```python
from build123d import *

# Parameters (mm, degrees)
BOSS_EXTRUDE1_DEPTH  = 2.5
FILLET1_R            = 5
BOSS_EXTRUDE2_DEPTH  = 9.8
CUT_EXTRUDE1_DEPTH   = 9.8
CUT_EXTRUDE2_DEPTH   = 89.657557489
BOSS_EXTRUDE3_DEPTH  = 11.7
MIRROR4_COPY_1_DEPTH = 11.7
SKETCH8_W            = 22.2
SKETCH8_H            = 28.2
CUT_EXTRUDE3_DEPTH   = 10


with BuildPart() as part:
    # Sketch1 → Boss-Extrude1 (new body)
    with BuildSketch(Plane(origin=(0, 0, 0), x_dir=(1, 0, 0), z_dir=(0, 1, 0))):
        with BuildLine():
            Line((-46.5, 30), (46.5, 30))
            ThreePointArc((46.5, 30), (50.035533906, 28.535533906), (51.5, 25))
            Line((51.5, 25), (51.5, -25))
            ThreePointArc((51.5, -25), (50.035533906, -28.535533906), (46.5, -30))
            Line((46.5, -30), (-46.5, -30))
            ThreePointArc((-46.5, -30), (-50.035533906, -28.535533906), (-51.5, -25))
            Line((-51.5, -25), (-51.5, 25))
            ThreePointArc((-51.5, 25), (-50.035533906, 28.535533906), (-46.5, 30))
        make_face()
    extrude(amount=BOSS_EXTRUDE1_DEPTH)

    # Fillet1
    # the kernel refuses this fillet: 5 mm, written as the material it takes off along each edge
    with BuildSketch(Plane(origin=(-46.5, 2.5, -25), x_dir=(-1, 0, 0), z_dir=(0, 0, 1))) as fillet1_piece_1:
        with BuildLine():
            CenterArc((0.669872981, 5), FILLET1_R, 270, 60)
            Line((0.669872981, 0), (0.669872981, -0.1))
            Line((0.669872981, -0.1), (5, -0.1))
            Line((5, -0.1), (5.1, 0))
            ThreePointArc((5.1, 0), (5.1, 1.25), (5.08660254, 2.45))
            Line((5.08660254, 2.45), (5, 2.5))
        make_face()
    revolve(axis=Axis((-46.5, 2.5, -25), (0, -1, 0)), revolution_arc=90, mode=Mode.SUBTRACT)
    with BuildSketch(Plane(origin=(-46.5, 2.5, -30), x_dir=(0, -1, 0), z_dir=(1, 0, 0)), Plane(origin=(46.5, 2.5, 30), x_dir=(0, -1, 0), z_dir=(-1, 0, 0))) as fillet1_piece_2:
        with BuildLine():
            CenterArc((5, -4.330127019), FILLET1_R, 120, 60)
            Line((0, -4.330127019), (-0.1, -4.330127019))
            Line((-0.1, -4.330127019), (-0.1, 0))
            Line((-0.1, 0), (0, 0.1))
            ThreePointArc((0, 0.1), (1.25, 0.1), (2.45, 0.08660254))
            Line((2.45, 0.08660254), (2.5, 0))
        make_face()
    extrude(amount=93, mode=Mode.SUBTRACT)
    with BuildSketch(Plane(origin=(46.5, 2.5, -25), x_dir=(0, 0, -1), z_dir=(-1, 0, 0))) as fillet1_piece_3:
        with BuildLine():
            CenterArc((0.669872981, 5), FILLET1_R, 270, 60)
            Line((0.669872981, 0), (0.669872981, -0.1))
            Line((0.669872981, -0.1), (5, -0.1))
            Line((5, -0.1), (5.1, 0))
            ThreePointArc((5.1, 0), (5.1, 1.25), (5.08660254, 2.45))
            Line((5.08660254, 2.45), (5, 2.5))
        make_face()
    revolve(axis=Axis((46.5, 2.5, -25), (0, -1, 0)), revolution_arc=90, mode=Mode.SUBTRACT)
    with BuildSketch(Plane(origin=(51.5, 2.5, -25), x_dir=(0, -1, 0), z_dir=(0, 0, 1)), Plane(origin=(-51.5, 2.5, 25), x_dir=(0, -1, 0), z_dir=(0, 0, -1))) as fillet1_piece_4:
        with BuildLine():
            CenterArc((5, -4.330127019), FILLET1_R, 120, 60)
            Line((0, -4.330127019), (-0.1, -4.330127019))
            Line((-0.1, -4.330127019), (-0.1, 0))
            Line((-0.1, 0), (0, 0.1))
            ThreePointArc((0, 0.1), (1.25, 0.1), (2.45, 0.08660254))
            Line((2.45, 0.08660254), (2.5, 0))
        make_face()
    extrude(amount=50, mode=Mode.SUBTRACT)
    with BuildSketch(Plane(origin=(46.5, 2.5, 25), x_dir=(1, 0, 0), z_dir=(0, 0, -1))) as fillet1_piece_5:
        with BuildLine():
            CenterArc((0.669872981, 5), FILLET1_R, 270, 60)
            Line((0.669872981, 0), (0.669872981, -0.1))
            Line((0.669872981, -0.1), (5, -0.1))
            Line((5, -0.1), (5.1, 0))
            ThreePointArc((5.1, 0), (5.1, 1.25), (5.08660254, 2.45))
            Line((5.08660254, 2.45), (5, 2.5))
        make_face()
    revolve(axis=Axis((46.5, 2.5, 25), (0, -1, 0)), revolution_arc=90, mode=Mode.SUBTRACT)
    with BuildSketch(Plane(origin=(-46.5, 2.5, 25), x_dir=(0, 0, 1), z_dir=(1, 0, 0))) as fillet1_piece_6:
        with BuildLine():
            CenterArc((0.669872981, 5), FILLET1_R, 270, 60)
            Line((0.669872981, 0), (0.669872981, -0.1))
            Line((0.669872981, -0.1), (5, -0.1))
            Line((5, -0.1), (5.1, 0))
            ThreePointArc((5.1, 0), (5.1, 1.25), (5.08660254, 2.45))
            Line((5.08660254, 2.45), (5, 2.5))
        make_face()
    revolve(axis=Axis((-46.5, 2.5, 25), (0, -1, 0)), revolution_arc=90, mode=Mode.SUBTRACT)

    # Sketch2 → Boss-Extrude2 (add)
    with BuildSketch(Plane.XZ):
        Polygon((-36.2, 28.5), (-24.5, 28.5), (-24.5, 26.5), (-29.35, 26.5), (-29.35, 20.5), (-31.35, 20.5), (-31.35, 26.5), (-36.2, 26.5), align=None)
        Polygon((48.225, -3.282847821), (46.225, -3.282847821), (46.225, -0.999790058), (40.225, -0.999790058), (40.225, 1), (46.225, 1), (46.225, 3.417152179), (48.225, 3.417152179), align=None)
        Polygon((24.5, 28.5), (36.2, 28.5), (36.2, 26.5), (31.35, 26.5), (31.35, 20.5), (29.35, 20.5), (29.35, 26.5), (24.5, 26.5), align=None)
        Polygon((24.5, -26.5), (29.35, -26.5), (29.35, -20.5), (31.35, -20.5), (31.35, -26.5), (36.2, -26.5), (36.2, -28.5), (24.5, -28.5), align=None)
        Polygon((-36.2, -28.5), (-24.5, -28.5), (-24.5, -26.5), (-29.35, -26.5), (-29.35, -20.5), (-31.35, -20.5), (-31.35, -26.5), (-36.2, -26.5), align=None)
        Polygon((-48.225, 3.417152179), (-46.225, 3.417152179), (-46.225, 1), (-40.225, 1), (-40.225, -0.999790058), (-46.225, -0.999790058), (-46.225, -3.282847821), (-48.225, -3.282847821), align=None)
    extrude(amount=BOSS_EXTRUDE2_DEPTH)

    # Sketch4 → Cut-Extrude1 (cut)
    with BuildSketch(Plane(origin=(0, 0, -0.999790058), x_dir=(-1, 0, 0), z_dir=(0, 0, -1))):
        Polygon((40.225, 0), (46.225, -9.8), (40.225, -9.8), align=None)
    cut_extrude1 = extrude(amount=-CUT_EXTRUDE1_DEPTH, mode=Mode.SUBTRACT)

    # Mirror1: Cut-Extrude1 across plane
    add(cut_extrude1.mirror(Plane(origin=(0, 0, 0), x_dir=(0, 0, 1), z_dir=(1, 0, 0))), mode=Mode.SUBTRACT)

    # Sketch5 → Cut-Extrude2 (cut, through all)
    with BuildSketch(Plane.ZY.offset(31.35)):
        Polygon((-26.5, -9.8), (-20.5, 0), (-20.5, -9.8), align=None)
    cut_extrude2 = extrude(amount=-CUT_EXTRUDE2_DEPTH, mode=Mode.SUBTRACT)

    # Mirror2: Cut-Extrude2 across plane
    add(cut_extrude2.mirror(Plane.XY), mode=Mode.SUBTRACT)

    # Sketch6 → Boss-Extrude3 (add)
    with BuildSketch(Plane(origin=(36.2, 0, 0), x_dir=(0, 0, -1), z_dir=(1, 0, 0))):
        Polygon((-28.5, -3), (-28.5, -7.5), (-30, -3.726144837), align=None)
    boss_extrude3 = extrude(amount=-BOSS_EXTRUDE3_DEPTH)

    # Mirror3: Boss-Extrude3 across plane
    add(boss_extrude3.mirror(Plane(origin=(0, 0, 0), x_dir=(0, 0, 1), z_dir=(1, 0, 0))))

    # Mirror4: Boss-Extrude3 across plane
    add(boss_extrude3.mirror(Plane.XY))

    # Mirror4 copy 1 sketch → Mirror4 copy 1 (add)
    with BuildSketch(Plane.ZY.offset(36.2)):
        Polygon((-28.5, -3), (-28.5, -7.5), (-30, -3.726144837), align=None)
    extrude(amount=-MIRROR4_COPY_1_DEPTH)

    # Sketch8 → Cut-Extrude3 (cut)
    with BuildSketch(Plane.XZ):
        with Locations((-21.1, 0)):
            Rectangle(SKETCH8_W, SKETCH8_H)
        with Locations((21.1, 0)):
            Rectangle(SKETCH8_W, SKETCH8_H)
    extrude(amount=-CUT_EXTRUDE3_DEPTH, mode=Mode.SUBTRACT)


solid = part.part
```
Check sheet for the modelled part. Datum: model origin and axes. Units: mm. A direction names the side the tool comes from. Round coordinates to 2 decimals unless told otherwise and drop trailing zeros. Order: outer loops, then holes, each group sorted by start corner. A loop starts at its lowest first (then second) coordinate and runs counter-clockwise, first axis right, second up. Notation, with made-up numbers: M -22.5,89 L 5.5,89 A18 ccw 5.5,99 Z; hole C -23,29 d8. An arc over 180 degrees is marked long. Answer in a Markdown table with one row per item.
(1) Set-up check for faces 4 (the flat face through (31.35, -3, -25)), 5 (the flat face through (-44, -4, 1)), 6 (the flat face through (30, -1, -28.5)), 7 (the flat face through (24.5, -5, 28)): record each of +Z, -Z, +X, -X, +Y, -Y from which the full face is reachable in a straight line by a thin tool's end or side.
Findings:
| item | result |
|---|---|
| face 4 | +X, -Y |
| face 5 | +Z, -Y |
| face 6 | -Z, +X, -X |
| face 7 | +Z, -Z, -Y |
(2) Section check D-D on y = -5.5. Give the number of separate pieces and of enclosed holes in the cut face, plus the area to 3 significant figures.
Findings:
| item | result |
|---|---|
| separate pieces | 6 |
| enclosed holes | 0 |
| area | 189 mm^2 |
(3) Section check C-C on x = 35. Record the boundary of the cut face in (y, z).
Findings:
| item | result |
|---|---|
| outline | M -9.8,-28.5 L -7.5,-28.5 L -3.73,-30 L -3,-28.5 L 0,-28.5 L 0,-30 A5 ccw 2.5,-25.67 L 2.5,25.67 A5 ccw 0,30 L 0,28.5 L -3,28.5 L -3.73,30 L -7.5,28.5 L -9.8,28.5 L -9.8,26.5 L 0,26.5 L 0,-26.5 L -9.8,-26.5 Z |
(4) Section check B-B on x = -17. Record the boundary of the cut face in (y, z).
Findings:
| item | result |
|---|---|
| outline | M 0,-30 A5 ccw 2.5,-25.67 L 2.5,-14.1 L 0,-14.1 Z; M 0,14.1 L 2.5,14.1 L 2.5,25.67 A5 ccw 0,30 Z |
(5) Gauge pin test, flat ends, axial feed: pin 1 (0.8 mm diameter, centred on y = 1, z = -7, fed in from +X); pin 2 (5.5 mm diameter, centred on x = -26, y = -6.5, fed in from -Z); pin 3 (5 mm diameter, centred on y = 0.5, z = 3.5, fed in from -X). Record the tip position at first contact, or that the pin passes through.
Findings:
| item | result |
|---|---|
| pin 1 | stops at x = 51.09 |
| pin 2 | stops at z = -29.99 |
| pin 3 | stops at x = -51.5 |
(6) Section check A-A on z = 7. Record the boundary of the cut face in (x, y).
Findings:
| item | result |
|---|---|
| outline | M -51.5,0 L -32.2,0 L -32.2,2.5 L -47.17,2.5 A5 ccw Z; M -10,0 L 10,0 L 10,2.5 L -10,2.5 Z; M 32.2,0 L 51.5,0 A5 ccw 47.17,2.5 L 32.2,2.5 Z |
(7) Material ranges on line 1 along X through (y, z) = (-6.5, 27); line 2 along X through (y, z) = (1, 4); line 3 along X through (y, z) = (-2.25, -22), recorded low to high. Write a range as from..to.
Findings:
| item | result |
|---|---|
| line 1 | x = -36.2..-24.5, 24.5..36.2 |
| line 2 | x = -50.74..-32.2, -10..10, 32.2..50.74 |
| line 3 | x = -31.35..-29.35, 29.35..31.35 |
(8) Draft check along Y on faces 1 (the flat face through (30, -1, 28.5)), 2 (the flat face through (30.336, -4.969, -23.542)), 3 (the flat face through (-34, -5, -26.5)). Enter one of: +Y half, -Y half, draft (parallel to the pull), parting line (faces both ways), or undercut.
Findings:
| item | result |
|---|---|
| face 1 | undercut |
| face 2 | -Y half |
| face 3 | draft |
